Check sheet for the modelled part. Datum: model origin and axes. Units: mm. A direction names the side the tool comes from. Coordinates: 2 decimals unless noted, no trailing zeros. Write each loop counter-clockwise with the first axis right and the second up, starting at its lowest first coordinate (ties: lowest second). Pieces come first, ordered by that corner, then holes. Notation, with made-up numbers: (78.25, -15) - (133.25, -15) arc R16 cw to (133.25, -11) - close; hole circle Ø3 at (63, 12.25). An arc over 180 degrees is marked (long way). Use one line per item in the form item = value. Start each with the question number.
1. Go/stop test with flat-tipped pins: pin 1 Ø3 at (x, y) = (8.5, 2) entering from +Z; pin 2 Ø4 at (x, y) = (-0.5, -4.5) entering from -Z; pin 3 Ø6 at (y, z) = (0, 2) entering from -X. Record where each tip stops, or that it passes through.
2. Cross-section at B-B on z = 0. Record the boundary of the cut face in (x, y), then the cut area to 3 significant figures.
3. Cross-section at A-A on y = 0. Record the boundary of the cut face in (x, z), then the cut area to 3 significant figures.
4. Scan lines: line 1 along Z through (x, y) = (0, -0.5); line 2 along X through (y, z) = (0, 0); line 3 along Z through (x, y) = (0, 1.5). Record each from-to range of solid material in increasing order.
5. Tool access check on faces 4 (the face through (-6, 0, 36)), 5 (the face through (9.043, -0.199, 15.964)). Record the directions out of +Z, -Z, +X, -X, +Y, -Y that give a thin tool (end or side, any length) a straight path to the whole face; none if there is none.
6. Cross-section at C-C on z = 42. Record the boundary of the cut face in (x, y), then the cut area to 3 significant figures.
7. Draft check along Z on faces 1 (the face through (-10.316, 0.084, 7.91)), 2 (the face through (0, 0, 54)), 3 (the face through (0, 6, 14)). Enter one of: +Z half, -Z half, draft (parallel to the pull), parting line (faces both ways), or undercut.
```python
from build123d import *

# Parameters (mm, degrees)
SZKIC1_W                        = 6
SZKIC1_H                        = 33
WYTNIJ_WYCI_GNI_CIE1_DEPTH      = 17
WYTNIJ_WYCI_GNI_CIE1_DEPTH_BACK = 17
SZKIC3_R                        = 13
WYTNIJ_WYCI_GNI_CIE2_DEPTH      = 7
WYTNIJ_WYCI_GNI_CIE2_DEPTH_BACK = 7
SFAZOWANIE1_SIZE                = 1.65


with BuildPart() as part:
    # Szkic1 → Obrót1 (revolve)
    with BuildSketch(Plane(origin=(0, 0, 0), x_dir=(1, 0, 0), z_dir=(0, 1, 0))):
        with BuildLine():
            Line((0, 16), (0, -21))
            Line((0, -21), (6, -21))
            Line((6, -21), (13.691822011, -8.278527045))
            ThreePointArc((13.691822011, -8.278527045), (13.936578359, 7.859502761), (0, 16))
        make_face()
        with Locations((3, -37.5)):
            Rectangle(SZKIC1_W, SZKIC1_H)
    revolve(axis=Axis((0, 0, -26.043516498), (0, 0, 1)))

    # Szkic2 → Wytnij-wyciągnięcie1 (cut, two sides)
    with BuildSketch(Plane(origin=(0, 0, 0), x_dir=(0, 0, -1), z_dir=(1, 0, 0))) as wytnij_wyci_gni_cie1_sk:
        with BuildLine():
            Line((-21, 6), (14.832396974, 6))
            ThreePointArc((14.832396974, 6), (5.052656155, 15.181260349), (-8.278527045, 13.691822011))
            Line((-8.278527045, 13.691822011), (-21, 6))
        make_face()
        with BuildLine():
            Line((-21, -6), (14.832396974, -6))
            ThreePointArc((14.832396974, -6), (5.052656155, -15.181260349), (-8.278527045, -13.691822011))
            Line((-8.278527045, -13.691822011), (-21, -6))
        make_face()
    extrude(amount=WYTNIJ_WYCI_GNI_CIE1_DEPTH, mode=Mode.SUBTRACT)
    extrude(wytnij_wyci_gni_cie1_sk.sketch, amount=-WYTNIJ_WYCI_GNI_CIE1_DEPTH_BACK, mode=Mode.SUBTRACT)

    # Szkic3 → Wytnij-wyciągnięcie2 (cut, two sides)
    with BuildSketch(Plane(origin=(0, 0, 0), x_dir=(1, 0, 0), z_dir=(0, 1, 0))) as wytnij_wyci_gni_cie2_sk:
        Circle(SZKIC3_R)
    extrude(amount=WYTNIJ_WYCI_GNI_CIE2_DEPTH, mode=Mode.SUBTRACT)
    extrude(wytnij_wyci_gni_cie2_sk.sketch, amount=-WYTNIJ_WYCI_GNI_CIE2_DEPTH_BACK, mode=Mode.SUBTRACT)

    # Sfazowanie1
    sfazowanie1_edges = [part.edges().sort_by_distance(p)[0] for p in [
        (-6, 0, 54),
    ]]
    chamfer(sfazowanie1_edges, length=SFAZOWANIE1_SIZE)


solid = part.part
```
Final values:
q1.pin_1 = 18.96
q1.pin_2 = -15.8
q1.pin_3 = -16
q2.outline = (-14.83, -6) - (-13, -6) - (-13, 6) - (-14.83, 6) arc R16 ccw to start; (13, -6) - (14.83, -6) arc R16 ccw to (14.83, 6) - (13, 6) - close
q2.area = 62.8 mm²
q3.outline = (-13.69, 8.28) arc R16 ccw (long way) to (13.69, 8.28) - (6, 21) - (6, 52.35) - (4.35, 54) - (-4.35, 54) - (-6, 52.35) - (-6, 21) - close; hole circle Ø26 at (0, 0)
q3.area = 768 mm²
q4.line_1 = -15.99 to -13, 13 to 54
q4.line_2 = -16 to -13, 13 to 16
q4.line_3 = -15.93 to -13, 13 to 54
q5.face_4 = +Z
q5.face_5 = +Z, +X
q6.outline = circle Ø12 at (0, 0)
q6.area = 113 mm²
q7.face_1 = undercut
q7.face_2 = +Z half
q7.face_3 = draft
